Verification items for this drawing (mm, ordinates from the low corner). Round coordinates to 2 decimals unless told otherwise and drop trailing zeros. Write each loop counter-clockwise with the first axis right and the second up, starting at its lowest first coordinate (ties: lowest second). Pieces come first, ordered by that corner, then holes. Notation, with made-up numbers: (4, -33.5) -> (28, -33.5) arc R24 cw to (28, -14.5) -> close; hole circle Ø2 at (-28, 53.25). An arc over 180 degrees is marked (long way). Use one line per item in the form item = value. Start each with the question number.
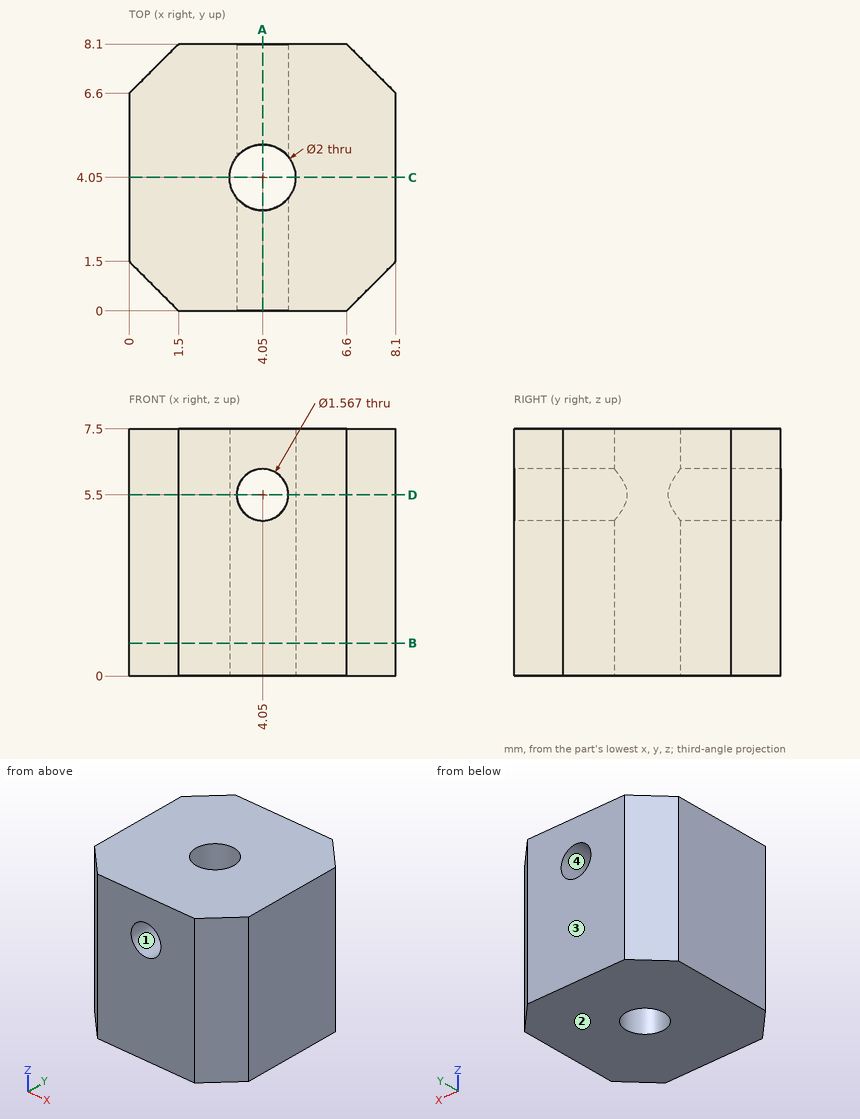
1. Sectioned sample at B-B (z = 1). Enter the section's corners in (x, y).
2. Sectioned sample at C-C (y = 4.05). Enter the section's corners in (x, z), and give its area (4 significant figures).
3. Sectioned sample at D-D (z = 5.5). Enter the section's corners in (x, y).
4. Depth check by flat-ended pin: pin 1 (0.9 mm diameter, centred on x = 4.05, z = 5.5, fed in from +Y). Enter the tip coordinate at first touch or a pass-through.
5. Mould release check, pull along Z, two halves, no side actions. Record for the marked faces 1, 2, 3 and 4: +Z half, -Z half, draft (parallel to the pull), parting line (faces both ways), or undercut.
6. Sectioned sample at A-A (x = 4.05). Enter the section's corners in (y, z).
7. Scan lines: probe 1 along X at (y, z) = (6.45, 5.5); probe 2 along Y at (x, z) = (4.05, 4). Record each from-to range of solid material in increasing order.
Returned:
q1.outline = (0, 1.5) -> (1.5, 0) -> (6.6, 0) -> (8.1, 1.5) -> (8.1, 6.6) -> (6.6, 8.1) -> (1.5, 8.1) -> (0, 6.6) -> close; hole circle Ø2 at (4.05, 4.05)
q2.outline = (0, 0) -> (3.05, 0) -> (3.05, 7.5) -> (0, 7.5) -> close; (5.05, 0) -> (8.1, 0) -> (8.1, 7.5) -> (5.05, 7.5) -> close
q2.area = 45.75 mm^2
q3.outline = (0, 1.5) -> (1.5, 0) -> (3.27, 0) -> (3.27, 3.43) arc R1 cw to (3.27, 4.67) -> (3.27, 8.1) -> (1.5, 8.1) -> (0, 6.6) -> close; (4.83, 0) -> (6.6, 0) -> (8.1, 1.5) -> (8.1, 6.6) -> (6.6, 8.1) -> (4.83, 8.1) -> (4.83, 4.67) arc R1 cw to (4.83, 3.43) -> close
q4.pin_1 = through
q5.face_1 = undercut
q5.face_2 = -Z half
q5.face_3 = draft
q5.face_4 = undercut
q6.outline = (0, 0) -> (3.05, 0) -> (3.05, 4.72) -> (0, 4.72) -> close; (0, 6.28) -> (3.05, 6.28) -> (3.05, 7.5) -> (0, 7.5) -> close; (5.05, 0) -> (8.1, 0) -> (8.1, 4.72) -> (5.05, 4.72) -> close; (5.05, 6.28) -> (8.1, 6.28) -> (8.1, 7.5) -> (5.05, 7.5) -> close
q7.probe_1 = 0 to 3.27, 4.83 to 8.1
q7.probe_2 = 0 to 3.05, 5.05 to 8.1
